from build123d import *

# Parameters (mm, degrees)
F0_W         = 40
F0_H         = 70
F1_DEPTH     = 7
F2_R         = 5
F3_R         = 2.0663885281
F4_DEPTH     = 5
F5_T1_DEPTH  = 60
F5_T3_DEPTH  = 30
F5_T6_ANGLE  = 90
F5_T8_ANGLE  = 90
F5_T10_ANGLE = 90
F5_T12_ANGLE = 90
F5_T14_ANGLE = 90
F5_T16_ANGLE = 90
F5_T18_ANGLE = 90
F5_T20_ANGLE = 90
F6_R         = 3.1424887648
F7_DEPTH     = 1


# Not quite as in the source:
# - a fillet or chamfer that OpenCascade refuses, or shapes differently, is made with other operations: its cross-section is extruded or revolved along the edge and cut away or added


with BuildPart() as f1:
    # F0 (on Top) → F1 (new body)
    with BuildSketch(Plane.XY):
        with Locations((20, 35)):
            Rectangle(F0_W, F0_H)
    extrude(amount=F1_DEPTH)

    # F2
    f2_edges = [f1.edges().sort_by_distance(p)[0] for p in [
        (40, 0, 3.5),
        (40, 70, 3.5),
        (0, 0, 3.5),
        (0, 70, 3.5),
    ]]
    fillet(f2_edges, radius=F2_R)

    # F3 (on face) → F4 (cut)
    with BuildSketch(Plane(origin=(0, 70, 0), x_dir=(-1, 0, 0), z_dir=(0, 1, 0))):
        with Locations((-29.0856193751, 3.5)):
            Circle(F3_R)
    extrude(amount=-F4_DEPTH, mode=Mode.SUBTRACT)

    # F5: fillet of radius 2 on 16 edges, made by hand

    # F5_s2 → F5_t1 (cut)
    with BuildSketch(Plane.XZ.offset(-65)):
        with BuildLine():
            ThreePointArc((2, 7), (0.5857864376, 6.4142135624), (0, 5))
            Line((0, 5), (0, 7))
            Line((0, 7), (2, 7))
        make_face()
        with BuildLine():
            ThreePointArc((2, 0), (0.5857864376, 0.5857864376), (0, 2))
            Line((0, 2), (0, 0))
            Line((0, 0), (2, 0))
        make_face()
        with BuildLine():
            ThreePointArc((38, 0), (39.4142135624, 0.5857864376), (40, 2))
            Line((40, 2), (40, 0))
            Line((40, 0), (38, 0))
        make_face()
        with BuildLine():
            ThreePointArc((38, 7), (39.4142135624, 6.4142135624), (40, 5))
            Line((40, 5), (40, 7))
            Line((40, 7), (38, 7))
        make_face()
    extrude(amount=F5_T1_DEPTH, mode=Mode.SUBTRACT)

    # F5_s4 → F5_t3 (cut)
    with BuildSketch(Plane.YZ.offset(5)):
        with BuildLine():
            ThreePointArc((70, 2), (69.4142135624, 0.5857864376), (68, 0))
            Line((68, 0), (70, 0))
            Line((70, 0), (70, 2))
        make_face()
        with BuildLine():
            ThreePointArc((70, 5), (69.4142135624, 6.4142135624), (68, 7))
            Line((68, 7), (70, 7))
            Line((70, 7), (70, 5))
        make_face()
        with BuildLine():
            ThreePointArc((2, 0), (0.5857864376, 0.5857864376), (0, 2))
            Line((0, 2), (0, 0))
            Line((0, 0), (2, 0))
        make_face()
        with BuildLine():
            ThreePointArc((2, 7), (0.5857864376, 6.4142135624), (0, 5))
            Line((0, 5), (0, 7))
            Line((0, 7), (2, 7))
        make_face()
    extrude(amount=F5_T3_DEPTH, mode=Mode.SUBTRACT)

    # F5_s5 → F5_t6 (revolve, cut)
    with BuildSketch(Plane.YZ.offset(35)):
        with BuildLine():
            ThreePointArc((68, 0), (69.4142135624, 0.5857864376), (70, 2))
            Line((70, 2), (70, 0))
            Line((70, 0), (68, 0))
        make_face()
    revolve(axis=Axis((35, 65, 0), (0, 0, -1)), revolution_arc=F5_T6_ANGLE, mode=Mode.SUBTRACT)

    # F5_s7 → F5_t8 (revolve, cut)
    with BuildSketch(Plane.YZ.offset(5)):
        with BuildLine():
            ThreePointArc((68, 0), (69.4142135624, 0.5857864376), (70, 2))
            Line((70, 2), (70, 0))
            Line((70, 0), (68, 0))
        make_face()
    revolve(axis=Axis((5, 65, 0), (0, 0, 1)), revolution_arc=F5_T8_ANGLE, mode=Mode.SUBTRACT)

    # F5_s9 → F5_t10 (revolve, cut)
    with BuildSketch(Plane.YZ.offset(35)):
        with BuildLine():
            ThreePointArc((2, 0), (0.5857864376, 0.5857864376), (0, 2))
            Line((0, 2), (0, 0))
            Line((0, 0), (2, 0))
        make_face()
    revolve(axis=Axis((35, 5, 0), (0, 0, 1)), revolution_arc=F5_T10_ANGLE, mode=Mode.SUBTRACT)

    # F5_s11 → F5_t12 (revolve, cut)
    with BuildSketch(Plane.XZ.offset(-5)):
        with BuildLine():
            ThreePointArc((2, 0), (0.5857864376, 0.5857864376), (0, 2))
            Line((0, 2), (0, 0))
            Line((0, 0), (2, 0))
        make_face()
    revolve(axis=Axis((5, 5, 0), (0, 0, 1)), revolution_arc=F5_T12_ANGLE, mode=Mode.SUBTRACT)

    # F5_s13 → F5_t14 (revolve, cut)
    with BuildSketch(Plane.YZ.offset(35)):
        with BuildLine():
            ThreePointArc((70, 5), (69.4142135624, 6.4142135624), (68, 7))
            Line((68, 7), (70, 7))
            Line((70, 7), (70, 5))
        make_face()
    revolve(axis=Axis((35, 65, 7), (0, 0, -1)), revolution_arc=F5_T14_ANGLE, mode=Mode.SUBTRACT)

    # F5_s15 → F5_t16 (revolve, cut)
    with BuildSketch(Plane.YZ.offset(5)):
        with BuildLine():
            ThreePointArc((70, 5), (69.4142135624, 6.4142135624), (68, 7))
            Line((68, 7), (70, 7))
            Line((70, 7), (70, 5))
        make_face()
    revolve(axis=Axis((5, 65, 7), (0, 0, 1)), revolution_arc=F5_T16_ANGLE, mode=Mode.SUBTRACT)

    # F5_s17 → F5_t18 (revolve, cut)
    with BuildSketch(Plane.YZ.offset(35)):
        with BuildLine():
            ThreePointArc((2, 7), (0.5857864376, 6.4142135624), (0, 5))
            Line((0, 5), (0, 7))
            Line((0, 7), (2, 7))
        make_face()
    revolve(axis=Axis((35, 5, 7), (0, 0, 1)), revolution_arc=F5_T18_ANGLE, mode=Mode.SUBTRACT)

    # F5_s19 → F5_t20 (revolve, cut)
    with BuildSketch(Plane.XZ.offset(-5)):
        with BuildLine():
            ThreePointArc((2, 7), (0.5857864376, 6.4142135624), (0, 5))
            Line((0, 5), (0, 7))
            Line((0, 7), (2, 7))
        make_face()
    revolve(axis=Axis((5, 5, 7), (0, 0, 1)), revolution_arc=F5_T20_ANGLE, mode=Mode.SUBTRACT)

    # F6 (on face) → F7 (cut)
    with BuildSketch(Plane.XY.offset(7)):
        with Locations((20, 8.9777829126)):
            Circle(F6_R)
    extrude(amount=-F7_DEPTH, mode=Mode.SUBTRACT)


solid = f1.part
Could you check a few things on this model? Use its own coordinates, in mm. A direction names the side the tool comes from. Give positions to 0.01 mm unless a question says otherwise; leave off trailing zeros. Order: outer loops, then holes, each group sorted by start corner. A loop starts at its lowest first (then second) coordinate and runs counter-clockwise, first axis right, second up. Notation, with made-up numbers: M 47.5,30 L 67.5,30 A32 cw 67.5,67 Z; hole C 5.25,60.5 d11. An arc over 180 degrees is marked long. One line per question, with ' | ' between items.
1. I'm going to push a flat-ended pin straight in: pin 1 (3 mm diameter, centred on x = 19, y = 10, fed in from +Z). Where does the tip first touch, or does it pass through?
Results:
pin 1: z = 6
2. If I drill on line 1 (Y direction, x = 20, z = 6.75); line 2 (Y direction, x = 22.5, z = 6.5); line 3 (X direction, y = 64, z = 5.25), over which ranges is the centre line in solid material (lowest first)?
Results:
line 1: 1.03 to 5.84, 12.12 to 68.97 | line 2: 0.68 to 7.07, 10.88 to 69.32 | line 3: 0.02 to 39.98
3. We'd pull the mould along Y, two halves only. Please class faces 1 (the face through (38, 1, 4)), 2 (the face through (22.9, 7.77, 6.51)), 3 (the face through (39.4, 35.42, 0.57)): +Y half, -Y half, draft (parallel to the pull), parting line (faces both ways), or undercut.
Results:
face 1: -Y half | face 2: undercut | face 3: draft
4. I want a section at B-B (z = 3.5). List the corners of the cut face in (x, y) for me.
Results:
outline: M 0,5 A5 ccw 5,0 L 35,0 A5 ccw 40,5 L 40,65 A5 ccw 35,70 L 31.15,70 L 31.15,65 L 27.02,65 L 27.02,70 L 5,70 A5 ccw 0,65 Z
5. For faces 4 (the face through (0, 35, 3)), 5 (the face through (20, 9, 6)), 6 (the face through (29, 65, 4)), which set-ups out of +Z, -Z, +X, -X, +Y, -Y let a thin tool reach every point of the face, with its end or its side?
Results:
face 4: +Z, -Z, -X, +Y, -Y | face 5: +Z | face 6: +Y
6. I want a section at A-A (x = 20). List the corners of the cut face in (y, z) for me, and give its area (3 significant figures).
Results:
outline: M 0,2 A2 ccw 2,0 L 68,0 A2 ccw 70,2 L 70,5 A2 ccw 68,7 L 12.12,7 L 12.12,6 L 5.84,6 L 5.84,7 L 2,7 A2 ccw 0,5 Z | area: 480 mm²
